```python
from build123d import *
from build123d.topology import SkipClean

# Parameters (mm, degrees)
SKIZZE1_R                         = 10
AUFSATZ_LINEAR_AUSTRAGEN1_DEPTH   = 2
SKIZZE2_R                         = 30
AUFSATZ_LINEAR_AUSTRAGEN2_DEPTH   = 2
AUFSATZ_LINEAR_AUSTRAGEN3_DEPTH   = 2
AUFSATZ_LINEAR_AUSTRAGEN3_2_DEPTH = 2
SKIZZE4_R                         = 10
AUFSATZ_LINEAR_AUSTRAGEN4_DEPTH   = 2
AUFSATZ_LINEAR_START              = 3
AUFSATZ_LINEAR_AUSTRAGEN15_DEPTH  = 3
SKIZZE9_R                         = 10
SCHNITT_LINEAR_AUSTRAGEN1_DEPTH   = 10
AUFSATZ_LINEAR_AUSTRAGEN16_DEPTH  = 3


with BuildPart() as part:
    # Skizze1 → Aufsatz-Linear austragen1 (new body)
    with BuildSketch(Plane(origin=(0, 0, 0), x_dir=(1, 0, 0), z_dir=(0, 1, 0))):
        with Locations(Location((0, 0, 0), (0, 0, 270))):
            Circle(SKIZZE1_R)
    extrude(amount=-AUFSATZ_LINEAR_AUSTRAGEN1_DEPTH)

    # Skizze2 → Aufsatz-Linear austragen2 (add)
    with BuildSketch(Plane(origin=(0, 0, 0), x_dir=(1, 0, 0), z_dir=(0, 1, 0))):
        with Locations(Location((0, 0, 0), (0, 0, 270))):
            Circle(SKIZZE2_R)
    extrude(amount=AUFSATZ_LINEAR_AUSTRAGEN2_DEPTH)



with BuildPart() as body_2:
    # Skizze3 → Aufsatz-Linear austragen3 (new body)
    with BuildSketch(Plane.XZ.offset(2)):
        with BuildLine():
            Line((-7.071067812, 7.071067812), (-9.192388155, 9.192388155))
            ThreePointArc((-9.192388155, 9.192388155), (-13, 0), (-9.192388155, -9.192388155))
            Line((-9.192388155, -9.192388155), (-7.071067812, -7.071067812))
            ThreePointArc((-7.071067812, -7.071067812), (-10, 0), (-7.071067812, 7.071067812))
        make_face()
    extrude(amount=AUFSATZ_LINEAR_AUSTRAGEN3_DEPTH)


with BuildPart() as body_3:
    # Skizze3 → Aufsatz-Linear austragen3 2 (new body)
    with BuildSketch(Plane.XZ.offset(2)):
        with BuildLine():
            Line((7.071067812, 7.071067812), (9.192388155, 9.192388155))
            ThreePointArc((9.192388155, 9.192388155), (13, 0), (9.192388155, -9.192388155))
            Line((9.192388155, -9.192388155), (7.071067812, -7.071067812))
            ThreePointArc((7.071067812, -7.071067812), (10, 0), (7.071067812, 7.071067812))
        make_face()
    extrude(amount=AUFSATZ_LINEAR_AUSTRAGEN3_2_DEPTH)


with BuildPart() as part_1:
    add(part.part)

    add(body_2.part)  # Aufsatz-Linear austragen4 merges body 2

    add(body_3.part)  # Aufsatz-Linear austragen4 merges body 3
    # Skizze4 → Aufsatz-Linear austragen4 (add)
    with BuildSketch(Plane.XZ.offset(2)):
        with Locations(Location((0, 0, 0), (0, 0, 90))):
            Circle(SKIZZE4_R)
    extrude(amount=AUFSATZ_LINEAR_AUSTRAGEN4_DEPTH)

    # Skizze8 → Aufsatz-Linear austragen15 (add)
    with BuildSketch(Plane(origin=(0, -2, 0), x_dir=(1, 0, 0), z_dir=(0, 1, 0)).offset(AUFSATZ_LINEAR_START)):
        with BuildLine():
            Line((10.076521944, -8.213629254), (7.737557516, -6.334840462))
            ThreePointArc((7.737557516, -6.334840462), (7.413457608, -6.711232845), (7.071067812, -7.071067812))
            Line((7.071067812, -7.071067812), (9.192388155, -9.192388155))
            ThreePointArc((9.192388155, -9.192388155), (9.646875989, -8.714228804), (10.076521944, -8.213629254))
        make_face()
        with BuildLine():
            Line((-7.071067812, 7.071067812), (-9.192388155, 9.192388155))
            ThreePointArc((-9.192388155, 9.192388155), (-9.636776415, 8.725396284), (-10.057468336, 8.236949111))
            Line((-10.057468336, 8.236949111), (-7.732766819, 6.340687449))
            ThreePointArc((-7.732766819, 6.340687449), (-7.410920578, 6.714034271), (-7.071067812, 7.071067812))
        make_face()
    extrude(amount=-AUFSATZ_LINEAR_AUSTRAGEN15_DEPTH)

    # Skizze9 → Schnitt-Linear austragen1 (cut)
    with BuildSketch(Plane.XZ):
        with Locations((-21.176717953, -21.176717953)):
            Circle(SKIZZE9_R)
    extrude(amount=-SCHNITT_LINEAR_AUSTRAGEN1_DEPTH, mode=Mode.SUBTRACT)

    # Skizze10 → Aufsatz-Linear austragen16 (add)
    with SkipClean():  # the faces are left unmerged after this step: merging them gives an invalid solid
        with BuildSketch(Plane.XZ):
            with BuildLine():
                Line((12.75, 0), (13, 0))
                ThreePointArc((13, 0), (12.612939215, 3.148613086), (11.474805482, 6.109733149))
                Line((11.474805482, 6.109733149), (11.250587553, 5.998898209))
                ThreePointArc((11.250587553, 5.998898209), (12.369468285, 3.091723524), (12.75, 0))
            make_face()
            with BuildLine():
                Line((9.53531372, -8.464058852), (9.730797288, -8.620416703))
                ThreePointArc((9.730797288, -8.620416703), (11.761619744, -5.537535643), (12.843968796, -2.008099992))
                Line((12.843968796, -2.008099992), (12.596380081, -1.973248299))
                ThreePointArc((12.596380081, -1.973248299), (11.531939258, -5.438462739), (9.53531372, -8.464058852))
            make_face()
            with BuildLine():
                Line((-12.731858626, -0.017690555), (-12.981862864, -0.017690555))
                ThreePointArc((-12.981862864, -0.017690555), (-12.594944508, -3.166086381), (-11.45802615, -6.127423703))
                Line((-11.45802615, -6.127423703), (-11.233808221, -6.016588763))
                ThreePointArc((-11.233808221, -6.016588763), (-12.351470245, -3.109195987), (-12.731858626, -0.017690555))
            make_face()
            with BuildLine():
                Line((-9.526622279, 8.457212783), (-9.72209655, 8.613563198))
                ThreePointArc((-9.72209655, 8.613563198), (-11.751242737, 5.529465141), (-12.833641797, 1.999945719))
                Line((-12.833641797, 1.999945719), (-12.586053082, 1.965094027))
                ThreePointArc((-12.586053082, 1.965094027), (-11.521565497, 5.430393435), (-9.526622279, 8.457212783))
            make_face()
        extrude(amount=AUFSATZ_LINEAR_AUSTRAGEN16_DEPTH)


solid = part_1.part
```
Geometry: final body of the model. Coordinates: model frame, mm. A direction names the side the tool comes from. Round coordinates to 2 decimals unless told otherwise and drop trailing zeros. Order: outer loops, then holes, each group sorted by start corner. A loop starts at its lowest first (then second) coordinate and runs counter-clockwise, first axis right, second up. Notation, with made-up numbers: (1, -7) - (40, -7) arc R19 ccw to (40, 28) - close; hole circle Ø1 at (-9.5, 2.25). An arc over 180 degrees is marked (long way). Write item = value, one per line. Start each with the question number.
Q1. Cut plane A-A on y = -1.2. Return the cut outline in (x, z).
Q2. Pull-direction query (Z, two-part tool) for faces 1 (the cylindrical face through (-11.729, -0.986, 5.576)), 2 (the flat face through (0, -4, 0)), 3 (the flat face through (8.923, -0.986, 7.287)); classes: +Z half, -Z half, draft (parallel to the pull), parting line (faces both ways), or undercut.
Q3. Pin query (flat end, axial travel): pin 1 (1.5 mm diameter, centred on y = 0, z = 21, fed in from -X); pin 2 (1 mm diameter, centred on y = 0, z = -11.5, fed in from -X); pin 3 (3 mm diameter, centred on y = 1, z = 10.5, fed in from +X). Return the tip coordinate at first contact, or that it passes through.
Q4. Ray query, line 1 (Y direction, x = -10.5, z = 6); line 2 (Y direction, x = -3, z = 15.5); line 3 (X direction, y = -1.4, z = -9). Return the intervals inside material, ascending. Write a range as from..to.
Q5. Access query for faces 4 (the flat face through (-8.91, -0.99, -7.3)), 5 (the cylindrical face through (-12.34, -0.99, -3.15)), 6 (the flat face through (-8, -2, -8)), 7 (the flat face through (-8, -3, 8)). Directions: +Z, -Z, +X, -X, +Y, -Y. A direction counts if a zero-diameter tool reaches every point of the face in a straight line with its end or side. Return the directions, or none.
Q6. Cut plane B-B on x = 0. Return the cut outline in (y, z).
Q7. Cut plane D-D on x = -22. Return the cut outline in (y, z).
Q8. Cut plane C-C on z = 20. Return the cut outline in (x, y).
Outcome:
q1.outline = (-12.98, -0.02) arc R13.02 ccw to (-11.46, -6.13) - (-11.23, -6.02) arc R12.77 cw to (-12.73, -0.02) - close; (-12.83, 2) - (-12.59, 1.97) arc R12.78 cw to (-9.53, 8.46) - (-9.72, 8.61) arc R13.03 ccw to start; (-10.06, -8.24) arc R13 ccw to (-9.19, -9.19) - (-7.07, -7.07) arc R10 ccw to (7.74, 6.33) - (10.08, 8.21) arc R13 ccw to (9.19, 9.19) - (7.07, 7.07) arc R10 ccw to (-7.73, -6.34) - close; (9.54, -8.46) - (9.73, -8.62) arc R13 ccw to (12.84, -2.01) - (12.6, -1.97) arc R12.75 cw to start; (11.25, 6) arc R12.75 cw to (12.75, 0) - (13, 0) arc R13 ccw to (11.47, 6.11) - close
q2.face_1 = +Z half
q2.face_2 = draft
q2.face_3 = undercut
q3.pin_1 = -22.13
q3.pin_2 = -27.91
q3.pin_3 = 28.62
q4.line_1 = -4..-2, 0..2
q4.line_2 = 0..2
q4.line_3 = -9.38..-9, -4.36..4.36
q5.face_4 = -X
q5.face_5 = none
q5.face_6 = -Z, -Y
q5.face_7 = +Z, -Y
q6.outline = (-4, -10) - (0, -10) - (0, -30) - (2, -30) - (2, 30) - (0, 30) - (0, 10) - (-4, 10) - close
q7.outline = (0, -11.21) - (2, -11.21) - (2, 20.4) - (0, 20.4) - close
q8.outline = (-22.36, 0) - (22.36, 0) - (22.36, 2) - (-22.36, 2) - close
